Geometry: final body of the model. Coordinates: model frame, mm. Give positions to 0.01 mm unless a question says otherwise; leave off trailing zeros. Use CSV: the item, a comma, the result in double quotes.
```python
from build123d import *

# Parameters (mm, degrees)
SKETCH1_W                                 = 300
SKETCH1_H                                 = 400
BOSS_EXTRUDE1_DEPTH                       = 16
CSK_FOR_8_FLAT_HEAD_MACHINE_SCREW_2_COUNT = 2
CSK_FOR_8_FLAT_HEAD_MACHINE_SCREW_2_PITCH = 26
FILLET1_R                                 = 8


with BuildPart() as part:
    # Sketch1 → Boss-Extrude1 (new body)
    with BuildSketch(Plane(origin=(0, 0, 0), x_dir=(1, 0, 0), z_dir=(0, 1, 0))):
        Rectangle(SKETCH1_W, SKETCH1_H)
    extrude(amount=BOSS_EXTRUDE1_DEPTH)

    # Sketch8 → CSK for #8 Flat Head Machine Screw (100)1 (revolve, cut)
    with BuildSketch(Plane(origin=(100, 0, 140), x_dir=(0, 0, -1), z_dir=(1, 0, 0))):
        Polygon((0, 0), (0, 26.350674586), (2.2479, 25), (2.2479, 1.651767624), (4.2164, 0), align=None)
    csk_for_8_flat_head_machine_screw_100 = revolve(axis=Axis((100, -6.35, 140), (0, 1, 0)), mode=Mode.SUBTRACT)

    # CSK for _8 Flat Head Machine Screw _ 2: CSK for #8 Flat Head Machine Screw (100)1 ×2
    with Locations(*[(-i * CSK_FOR_8_FLAT_HEAD_MACHINE_SCREW_2_PITCH, 0, 0) for i in range(1, CSK_FOR_8_FLAT_HEAD_MACHINE_SCREW_2_COUNT)]):
        add(csk_for_8_flat_head_machine_screw_100, mode=Mode.SUBTRACT)

    # Mirror1: CSK for #8 Flat Head Machine Screw (100)1 across plane
    add(csk_for_8_flat_head_machine_screw_100.mirror(Plane.XY), mode=Mode.SUBTRACT)

    # Mirror1 copy 1 sketch → Mirror1 copy 1 (revolve, cut)
    with BuildSketch(Plane(origin=(74, 0, -140), x_dir=(0, 0, 1), z_dir=(1, 0, 0))):
        Polygon((0, 0), (0, -26.350674586), (2.2479, -25), (2.2479, -1.651767624), (4.2164, 0), align=None)
    revolve(axis=Axis((74, -6.35, -140), (0, -1, 0)), mode=Mode.SUBTRACT)

    # Fillet1
    fillet1_edges = [part.edges().sort_by_distance(p)[0] for p in [
        (-150, 16, 0),
        (-150, 0, 0),
    ]]
    fillet(fillet1_edges, radius=FILLET1_R - 0.0001)  # a hair under: the kernel refuses the full size


solid = part.part
```
1. Pin query (flat end, axial travel): pin 1 Ø7 at (x, z) = (74, -140) entering from -Y; pin 2 Ø6 at (x, z) = (74, 140) entering from -Y; pin 3 Ø2 at (x, z) = (94.5, -92) entering from -Y; pin 4 Ø4 at (y, z) = (11.5, -95) entering from -X. Return the tip coordinate at first contact, or that it passes through.
Answer:
pin 1,"y = 0.6"
pin 2,"y = 1.02"
pin 3,"y = 0"
pin 4,"x = -149.86"
2. Pull-direction query (Z, two-part tool) for faces 1 (the face through (-2, 8, 200)), 2 (the face through (-147.719, 2.406, -2.8)), 3 (the face through (73.29, 1.55, 137.74)); classes: +Z half, -Z half, draft (parallel to the pull), parting line (faces both ways), or undercut.
Answer:
face 1,"+Z half"
face 2,"draft"
face 3,"undercut"
3. Line query: line 1 (Z direction, x = 100, y = 10); line 2 (X direction, y = 8.5, z = -140); line 3 (X direction, y = 9, z = 140). Output: solid intervals per line, ascending.
Answer:
line 1,"-200 to -142.25, -137.75 to 137.75, 142.25 to 200"
line 2,"-149.98 to 71.75, 76.25 to 97.75, 102.25 to 150"
line 3,"-149.94 to 71.75, 76.25 to 97.75, 102.25 to 150"
